For this review, use the dimensioned drawing (mm, ordinates from the lowest corner) and the shaded views. A direction names the side the tool comes from. Coordinates: 2 decimals unless noted, no trailing zeros. Loops run counter-clockwise (first coordinate to the right, second up) from the corner with the lowest first, then second, coordinate; pieces in that order, holes last. Notation, with made-up numbers: (38.25, 77.5) - (66.25, 77.5) arc R15 ccw to (66.25, 88.5) - close; hole circle Ø7 at (-33, 52). An arc over 180 degrees is marked (long way). One line per item, written item: value. Start each with the question number.
1. Insertion check: P1, Ø12, axis at x = 95.5, y = 40, coming from the -Z side; P2, Ø17, axis at x = 18, z = 62.5, coming from the +Y side; P3, Ø7.5, axis at y = 27, z = 5, coming from the +X side; P4, Ø22, axis at x = 62, y = 29.5, coming from the -Z side. Each pin has a flat end and moves straight along its axis. Give the tip position at first contact, or say it passes through.
2. To check wall thickness, follow line 1 (X direction, y = 21, z = 74); line 2 (Y direction, x = 20, z = 23); line 3 (X direction, y = 8.5, z = 11). State the ranges of each line that lie inside material, in increasing order.
3. We need section B-B, the plane x = 105. Give the boundary of the cut face in (y, z), then the cut area to 3 significant figures.
4. We need section C-C, the plane y = 54. Give the boundary of the cut face in (x, z).
5. We need section D-D, the plane x = 38. Give the boundary of the cut face in (y, z), then the cut area to 3 significant figures.
6. Mouldability with a two-part tool opening along X and no side actions: class the marked faces 4, 5 and 6 as +X half, -X half, draft (parallel to the pull), parting line (faces both ways), or undercut.
7. For the marked faces 1, 2 and 3, list the 3-axis set-ups (+Z, -Z, +X, -X, +Y, -Y) from which the entire face can be reached by the end or side of a thin tool; tool diameter is ignored.
8. We need section A-A, the plane z = 8.5. Give the boundary of the cut face in (x, y), then the cut area to 3 significant figures.
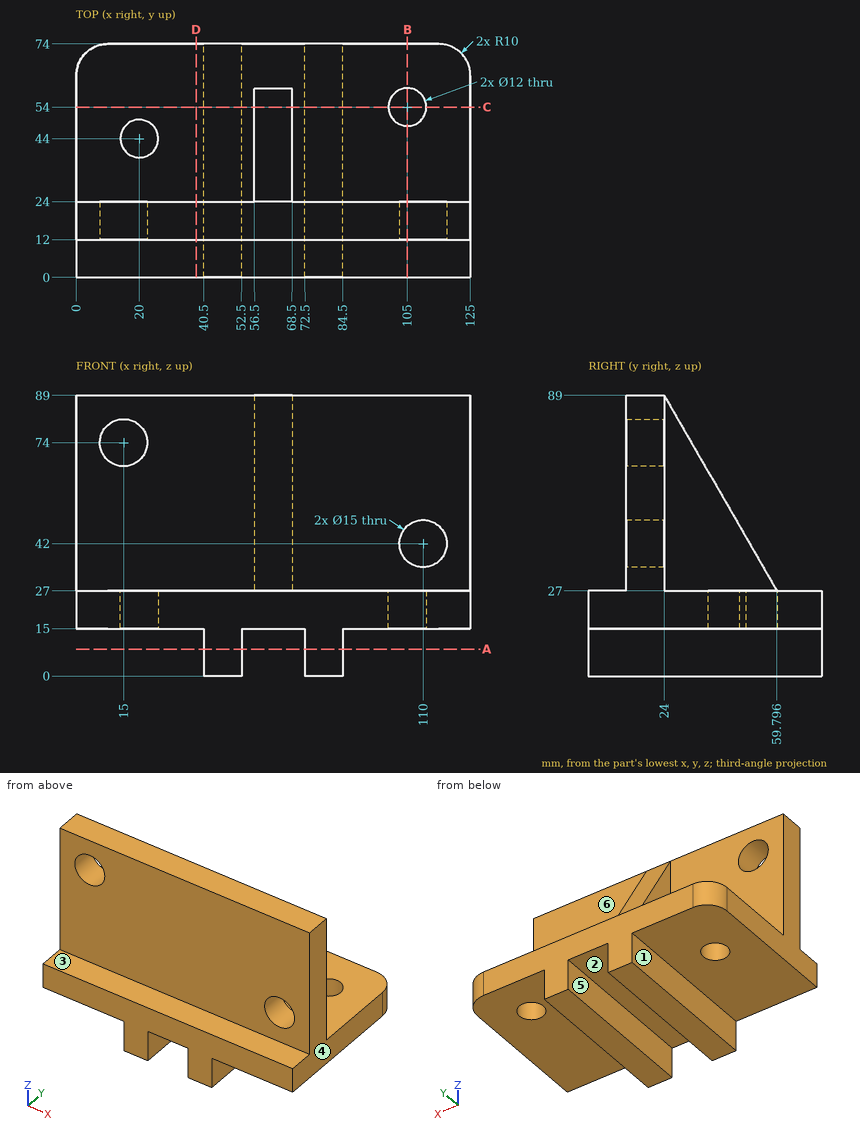
Findings below:
1. P1: z = 15
1. P2: y = 24
1. P3: x = 84.5
1. P4: z = 0
2. line 1: 0 to 7.5, 22.5 to 125
2. line 2: 0 to 38, 50 to 74
2. line 3: 40.5 to 52.5, 72.5 to 84.5
3. outline: (0, 15) - (48, 15) - (48, 27) - (24, 27) - (24, 36.41) - (12, 36.41) - (12, 27) - (0, 27) - close; (12, 47.59) - (24, 47.59) - (24, 89) - (12, 89) - close; (60, 15) - (74, 15) - (74, 27) - (60, 27) - close
3. area: 1,350 mm2
4. outline: (0, 15) - (40.5, 15) - (40.5, 0) - (52.5, 0) - (52.5, 15) - (72.5, 15) - (72.5, 0) - (84.5, 0) - (84.5, 15) - (99, 15) - (99, 27) - (68.5, 27) - (68.5, 37.04) - (56.5, 37.04) - (56.5, 27) - (0, 27) - close; (111, 15) - (125, 15) - (125, 27) - (111, 27) - close
5. outline: (0, 15) - (74, 15) - (74, 27) - (24, 27) - (24, 89) - (12, 89) - (12, 27) - (0, 27) - close
5. area: 1,630 mm2
6. face 4: +X half
6. face 5: undercut
6. face 6: draft
7. face 1: -Z, -X, +Y, -Y
7. face 2: -Z, +Y, -Y
7. face 3: +Z, +X, -X, -Y
8. outline: (40.5, 0) - (52.5, 0) - (52.5, 74) - (40.5, 74) - close; (72.5, 0) - (84.5, 0) - (84.5, 74) - (72.5, 74) - close
8. area: 1,780 mm2
